```python
from build123d import *

# Parameters (mm, degrees)
BOSS_EXTRUDE1_DEPTH = 218
CUT_EXTRUDE1_DEPTH  = 218
CUT_EXTRUDE2_DEPTH  = 218
SKETCH6_R           = 10
CUT_EXTRUDE3_DEPTH  = 218
SKETCH7_R           = 10
CUT_EXTRUDE4_DEPTH  = 218
CHAMFER1_SIZE       = 5


with BuildPart() as part:
    # Sketch1 → Boss-Extrude1 (new body)
    with BuildSketch(Plane(origin=(0, 0, 0), x_dir=(1, 0, 0), z_dir=(0, 1, 0))):
        with BuildLine():
            Line((8, -63), (13, -63))
            ThreePointArc((13, -63), (20.071067812, -65.928932188), (23, -73))
            Line((23, -73), (23, -155))
            Line((23, -155), (33, -155))
            Line((33, -155), (33, -65))
            ThreePointArc((33, -65), (24.205505282, -55.89329221), (21, -43.645843496))
            Line((21, -43.645843496), (21, 0))
            Line((21, 0), (0, 0))
            Line((0, 0), (0, -43.645843496))
            ThreePointArc((0, -43.645843496), (-3.205505282, -55.89329221), (-12, -65))
            Line((-12, -65), (-12, -155))
            Line((-12, -155), (-2, -155))
            Line((-2, -155), (-2, -100.45062745))
            Line((-2, -100.45062745), (-2, -73))
            ThreePointArc((-2, -73), (0.928932188, -65.928932188), (8, -63))
        make_face()
    extrude(amount=BOSS_EXTRUDE1_DEPTH)

    # Sketch3 → Cut-Extrude1 (cut)
    with BuildSketch(Plane.ZY):
        with BuildLine():
            ThreePointArc((25, 138.56265757), (35.089663756, 141.253339953), (43.645843496, 147.239396639))
            Line((43.645843496, 147.239396639), (43.645843496, 218))
            Line((43.645843496, 218), (0, 218))
            Line((0, 218), (0, 113.56265757))
            ThreePointArc((0, 113.56265757), (7.32233047, 131.2403271), (25, 138.56265757))
        make_face()
        with BuildLine():
            ThreePointArc((25, 88.56265757), (7.32233047, 95.884988041), (0, 113.56265757))
            Line((0, 113.56265757), (0, 0))
            Line((0, 0), (43.645843496, 0))
            Line((43.645843496, 0), (43.645843496, 79.885918501))
            ThreePointArc((43.645843496, 79.885918501), (35.089663756, 85.871975187), (25, 88.56265757))
        make_face()
    extrude(amount=-CUT_EXTRUDE1_DEPTH, mode=Mode.SUBTRACT)

    # Sketch5 → Cut-Extrude2 (cut)
    with BuildSketch(Plane.ZY.offset(12)):
        with BuildLine():
            ThreePointArc((66.899192484, 172.697482901), (72.753620331, 175.835761562), (79.282746191, 174.613618416))
            Line((79.282746191, 174.613618416), (140, 139.558495585))
            ThreePointArc((140, 139.558495585), (150.980762114, 128.577733471), (155, 113.577733471))
            Line((155, 113.577733471), (155, 218))
            Line((155, 218), (65, 218))
            Line((65, 218), (65, 170.618220852))
            Line((65, 170.618220852), (66.899192484, 172.697482901))
        make_face()
        Polygon((43.645843496, 147.239396639), (65, 170.618220852), (65, 218), (43.645843496, 218), align=None)
        Polygon((65, 0), (65, 58.531761997), (43.645843496, 79.885918501), (43.645843496, 0), align=None)
        with BuildLine():
            Line((155, 0), (155, 113.577733471))
            ThreePointArc((155, 113.577733471), (150.980762114, 98.577733471), (140, 87.596971358))
            Line((140, 87.596971358), (80.972769589, 53.163585587))
            Line((80.972769589, 53.163585587), (80.895268222, 53.11837536))
            ThreePointArc((80.895268222, 53.11837536), (74.5900063, 51.864180784), (68.824200411, 54.707561586))
            Line((68.824200411, 54.707561586), (65, 58.531761997))
            Line((65, 58.531761997), (65, 0))
            Line((65, 0), (155, 0))
        make_face()
    extrude(amount=-CUT_EXTRUDE2_DEPTH, mode=Mode.SUBTRACT)

    # Sketch6 → Cut-Extrude3 (cut)
    with BuildSketch(Plane(origin=(33, 0, 0), x_dir=(0, 0, -1), z_dir=(1, 0, 0))):
        with Locations((-125, 113.577733471)):
            Circle(SKETCH6_R)
    extrude(amount=-CUT_EXTRUDE3_DEPTH, mode=Mode.SUBTRACT)

    # Sketch7 → Cut-Extrude4 (cut)
    with BuildSketch(Plane(origin=(21, 0, 0), x_dir=(0, 0, -1), z_dir=(1, 0, 0))):
        with Locations((-25, 113.56265757)):
            Circle(SKETCH7_R)
    extrude(amount=-CUT_EXTRUDE4_DEPTH, mode=Mode.SUBTRACT)

    # Chamfer1
    chamfer1_edges = [part.edges().sort_by_distance(p)[0] for p in [
        (-12, 113.577733471, 135),
        (33, 113.577733471, 135),
        (0, 113.56265757, 35),
        (21, 113.56265757, 35),
    ]]
    chamfer(chamfer1_edges, length=CHAMFER1_SIZE)


solid = part.part
```
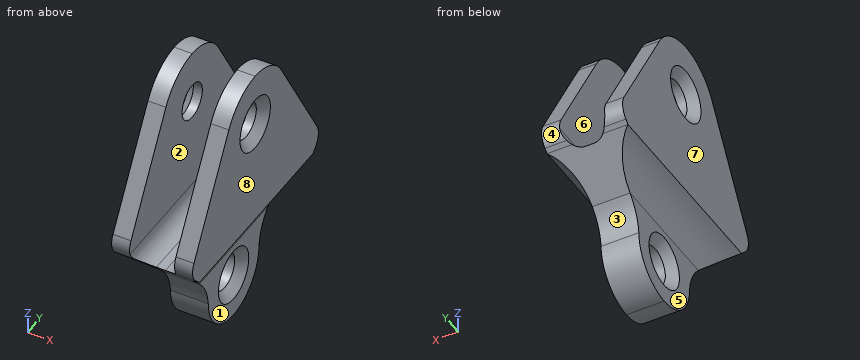
Could you check a few things on this model? Use its own coordinates, in mm. Face numbers are marked on the shaded views. A direction names the side the tool comes from. Round coordinates to 2 decimals unless told otherwise and drop trailing zeros. Loops run counter-clockwise (first coordinate to the right, second up) from the corner with the lowest first, then second, coordinate; pieces in that order, holes last. Notation, with made-up numbers: (7, -12) -> (65, -12) arc R9 ccw to (65, -5) -> close; hole circle Ø11 at (69, -4.75). An arc over 180 degrees is marked (long way). Put each result on its own line as item: value.
Q1. For pin 1 Ø1.5 at (y, z) = (129, 42) entering from -X; pin 2 Ø12 at (x, z) = (4.5, 77.5) entering from -Y; pin 3 Ø10 at (x, y) = (17, 91.5) entering from -Z; pin 4 Ø3 at (y, z) = (104, 32) entering from +X, each with a flat end and sliding along its axis, tell me the tip position at first contact or that it passes through.
Checks:
pin 1: x = 0
pin 2: through
pin 3: z = 6.73
pin 4: x = 19.35
Q2. Please list where these lines run through material, in increasing order: line 1 (X direction, y = 107, z = 93); line 2 (Y direction, x = 24.6, z = 125); line 3 (Z direction, x = 17, y = 154.5). Write a range as from..to.
Checks:
line 1: -12..-2, 23..33
line 2: 78.85..103.58, 123.58..148.22
line 3: 50.28..63.83
Q3. I want a section at B-B on z = 125. Write out the boundary of the cut face in (x, y).
Checks:
outline: (-12, 78.85) -> (-2, 78.85) -> (-2, 103.58) -> (-7, 103.58) -> (-12, 98.58) -> close; (-12, 128.58) -> (-7, 123.58) -> (-2, 123.58) -> (-2, 148.22) -> (-12, 148.22) -> close; (23, 78.85) -> (33, 78.85) -> (33, 98.58) -> (28, 103.58) -> (23, 103.58) -> close; (23, 123.58) -> (28, 123.58) -> (33, 128.58) -> (33, 148.22) -> (23, 148.22) -> close
Q4. Which directions (+Z, -Z, +X, -X, +Y, -Y) give clear straight access to the entire face, cutting with the end or side of a thin tool? Please do the marked faces 1, 2, 3, 4 and 5.
Checks:
face 1: -Z, +X, +Y, -Y
face 2: +Z, +Y, -Y
face 3: -Z, +X, -X, +Y
face 4: +X, -X, +Y
face 5: -Z, -X, +Y, -Y
Q5. I want a section at C-C on y = 63.5. Write out the boundary of the cut face in (x, z), and give its area (3 significant figures).
Checks:
outline: (-12, 65) arc R25 cw to (-6.12, 60.03) -> (27.12, 60.03) arc R25 cw to (33, 65) -> (33, 98.69) -> (23, 98.69) -> (23, 73) arc R10 cw to (13, 63) -> (8, 63) arc R10 cw to (-2, 73) -> (-2, 98.69) -> (-12, 98.69) -> close
area: 858 mm2
Q6. I want a section at A-A on x = 10. Write out the boundary of the cut face in (y, z).
Checks:
outline: (60.53, 63) -> (79.89, 43.65) arc R30 cw to (88.56, 25) arc R25 ccw to (138.56, 25) arc R30 cw to (147.24, 43.65) -> (168.43, 63) -> close; hole circle Ø20 at (113.56, 25)
Q7. I want a section at D-D on z = 107. Write out the boundary of the cut face in (x, y).
Checks:
outline: (-12, 68.35) -> (-2, 68.35) -> (-2, 158.61) -> (-12, 158.61) -> close; (23, 68.35) -> (33, 68.35) -> (33, 158.61) -> (23, 158.61) -> close
Q8. Thinking about a two-plate mould opening in X: for the marked faces 6, 7 and 8, which applies, pulls with the +X half, pulls with the -X half, needs draft (parallel to the pull), parting line crosses it, or undercut?
Checks:
face 6: undercut
face 7: pulls with the -X half
face 8: pulls with the +X half
